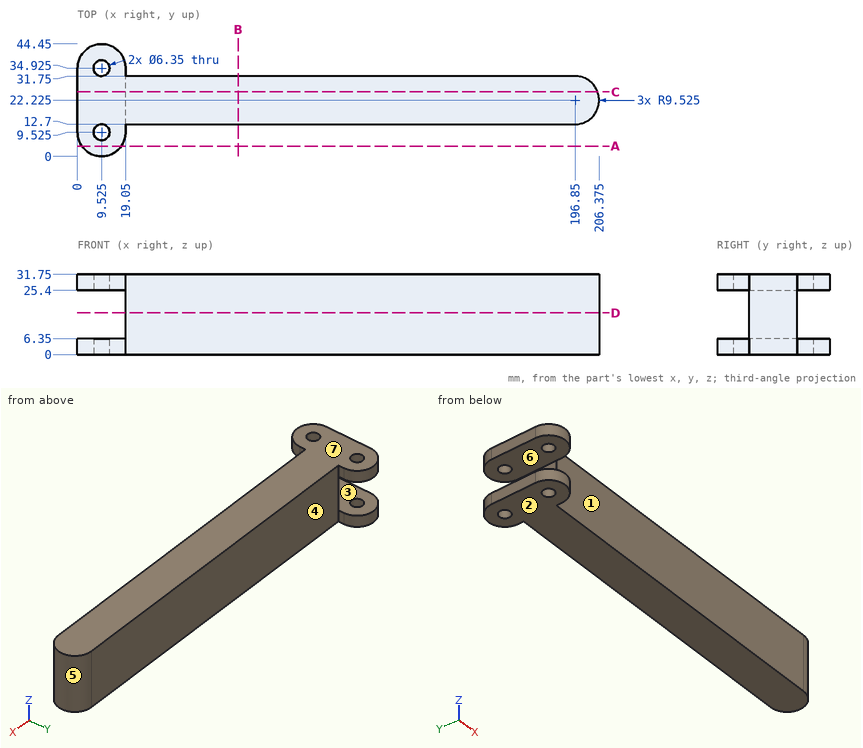
Drawing for the job (mm, zero at the part's lowest x, y, z). A direction names the side the tool comes from. Round coordinates to 2 decimals unless told otherwise and drop trailing zeros. Loops run counter-clockwise (first coordinate to the right, second up) from the corner with the lowest first, then second, coordinate; pieces in that order, holes last. Notation, with made-up numbers: (5.5, 87) - (19.5, 87) arc R21 ccw to (19.5, 91) - close; hole circle Ø9 at (-34.75, -12.5). An arc over 180 degrees is marked (long way). Return JSON: item names as keys, results as strings. Group by question number.
Q1. Band-saw the part on D-D on z = 16.5. Give the cut face in (x, y) (3 decimals).
Q2. Two-plate mould, pull along Z, no slides. Class the marked faces 5, 6 and 7: +Z half, -Z half, draft (parallel to the pull), parting line (faces both ways), or undercut.
Q3. Tool access for the marked faces 1, 2, 3 and 4: list every direction of +Z, -Z, +X, -X, +Y, -Y with a clear straight run to the whole face (end or side of a thin tool).
Q4. Flat gauge pins, fed straight in: pin 1 Ø9.5 at (y, z) = (18.5, 20) entering from -X; pin 2 Ø12 at (x, z) = (165.5, 18) entering from -Y; pin 3 Ø5.5 at (x, y) = (9.525, 9.525) entering from -Z (3 decimals); pin 4 Ø5 at (x, z) = (128.5, 18) entering from +Y. Where does each tip first touch, or does it go through?
Q5. Band-saw the part on C-C on y = 25.5. Give the cut face in (x, z).
Q6. Drill centre lines: line 1 along Z through (x, y) = (19, 16); line 2 along Y through (x, z) = (132, 14.5); line 3 along Y through (x, z) = (197.5, 13). Where is each one in solid material? Low to high. Write a range as [from, to].
Q7. Band-saw the part on A-A on y = 4. Give the cut face in (x, z), plus the area to 3 significant figures.
Q8. Band-saw the part on B-B on x = 63.5. Give the cut face in (y, z), plus the area to 3 significant figures.
Solutions:
{
 "1": {"outline": "(19.05, 12.7) - (196.85, 12.7) arc R9.525 ccw to (196.85, 31.75) - (19.05, 31.75) - close"},
 "2": {"face 5": "draft", "face 6": "undercut", "face 7": "+Z half"},
 "3": {"face 1": "+Z, -Z, +X, -Y", "face 2": "-Z, +X, -X, +Y, -Y", "face 3": "-X, +Y, -Y", "face 4": "+Z, -Z, +X, +Y"},
 "4": {"pin 1": "stops at x = 19.05", "pin 2": "stops at y = 12.7", "pin 3": "passes through", "pin 4": "stops at y = 31.75"},
 "5": {"outline": "(0, 0) - (205.79, 0) - (205.79, 31.75) - (0, 31.75) - (0, 25.4) - (19.05, 25.4) - (19.05, 6.35) - (0, 6.35) - close"},
 "6": {"line 1": "z = [0, 6.35], [25.4, 31.75]", "line 2": "y = [12.7, 31.75]", "line 3": "y = [12.72, 31.73]"},
 "7": {"outline": "(1.77, 0) - (17.28, 0) - (17.28, 6.35) - (1.77, 6.35) - close; (1.77, 25.4) - (17.28, 25.4) - (17.28, 31.75) - (1.77, 31.75) - close", "area": "197 mm^2"},
 "8": {"outline": "(12.7, 0) - (31.75, 0) - (31.75, 31.75) - (12.7, 31.75) - close", "area": "605 mm^2"}
}
